Geometry: see drawing. Coordinates: mm, zero at the bounding-box minimum. A direction names the side the tool comes from. Coordinates: 2 decimals unless noted, no trailing zeros. Write each loop counter-clockwise with the first axis right and the second up, starting at its lowest first coordinate (ties: lowest second). Pieces come first, ordered by that corner, then holes. Notation, with made-up numbers: (-11, 5) - (16, 5) arc R21 ccw to (16, 14) - close; hole circle Ø5 at (50.25, 75). An arc over 180 degrees is marked (long way). One line per question, with ' | ' between items. Start each with the question number.
1) Section query D-D on x = 3.6. Return loops of the section in (y, z).
2) Section query B-B on z = 2.95. Return loops of the section in (x, y).
3) Reachability of the marked faces 1, 2, 3, 4 and 5 from +Z, -Z, +X, -X, +Y, -Y: full face, straight path, thin tool, end or side. Return the list, or none.
4) Section query A-A on y = 6. Return loops of the section in (x, z), and give its area (3 significant figures).
5) Section query C-C on x = 1.8. Return loops of the section in (y, z).
6) First-contact query: P1, Ø0.5, axis at y = 2, z = 4, coming from the +X side; P2, Ø1.2, axis at x = 4, y = 5, coming from the -Z side; P3, Ø0.8, axis at x = 4, y = 3, coming from the +Z side. Flat tips, straight axial feed; report the tip coordinate or a pass-through.
7) Line query: line 1 (Y direction, x = 3, z = 4.05); line 2 (X direction, y = 0.5, z = 4.35). Output: solid intervals per line, ascending.
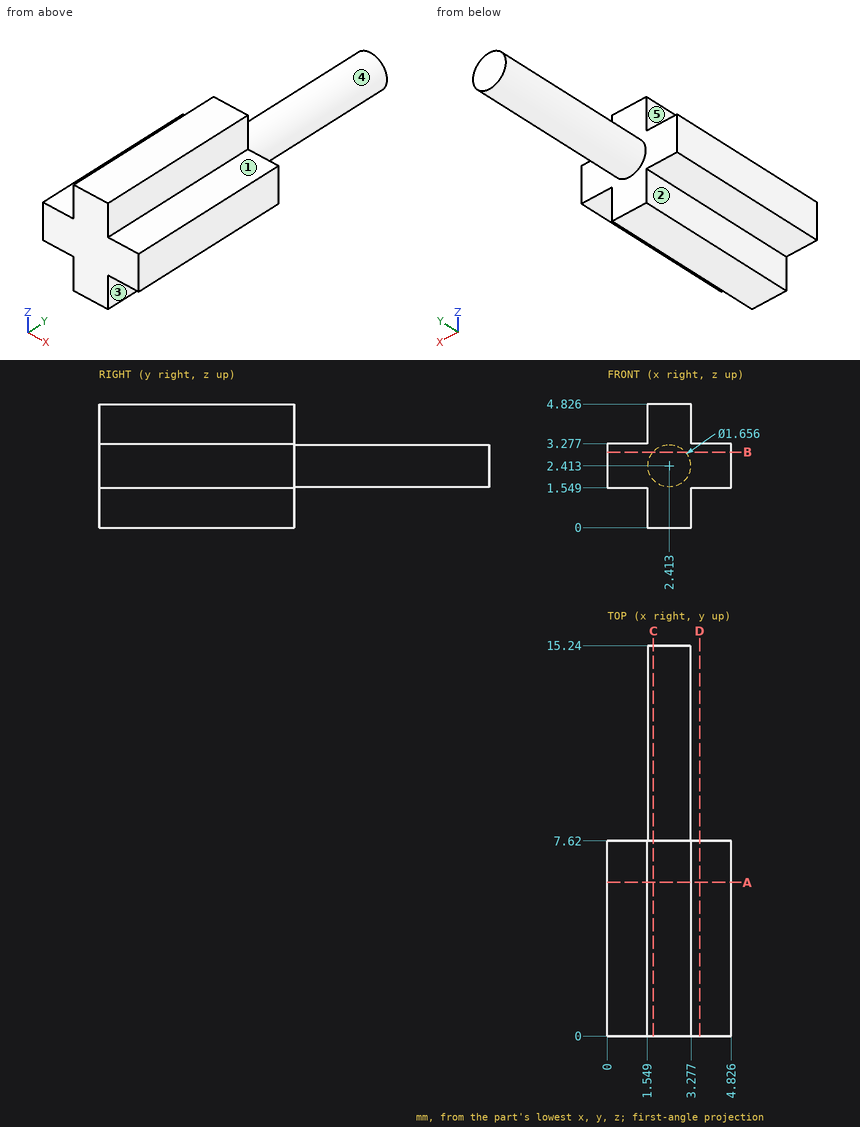
Answer key:
1) outline: (0, 1.55) - (7.62, 1.55) - (7.62, 3.28) - (0, 3.28) - close
2) outline: (0, 0) - (4.83, 0) - (4.83, 7.62) - (3.04, 7.62) - (3.04, 15.24) - (1.78, 15.24) - (1.78, 7.62) - (0, 7.62) - close
3) face 1: +Z, +X, +Y, -Y | face 2: -Z, -X, +Y, -Y | face 3: -Z, +X, +Y, -Y | face 4: +Y | face 5: +Z, -X, +Y, -Y
4) outline: (0, 1.55) - (1.55, 1.55) - (1.55, 0) - (3.28, 0) - (3.28, 1.55) - (4.83, 1.55) - (4.83, 3.28) - (3.28, 3.28) - (3.28, 4.83) - (1.55, 4.83) - (1.55, 3.28) - (0, 3.28) - close | area: 13.7 mm²
5) outline: (0, 0) - (7.62, 0) - (7.62, 1.86) - (15.24, 1.86) - (15.24, 2.97) - (7.62, 2.97) - (7.62, 4.83) - (0, 4.83) - close
6) P1: x = 3.28 | P2: z = 1.55 | P3: z = 3.28
7) line 1: 0 to 7.62 | line 2: 1.55 to 3.28
